```python
from build123d import *

# Parameters (mm, degrees)
SKETCH2_W               = 88.9
SKETCH2_H               = 152.4
BOSS_EXTRUDE1_DEPTH     = 5.9944
CUT_EXTRUDE2_DEPTH      = 177.535840076
CUT_EXTRUDE2_DEPTH_BACK = 177.535840076
SKETCH4_R               = 2.7305
BOSS_EXTRUDE2_DEPTH     = 101.6
FILLET1_R               = 3.81
FILLET2_R               = 2.54
BOSS_EXTRUDE3_DEPTH     = 20.32
FILLET3_R               = 3.81
FILLET6_R               = 3.81
FILLET7_R               = 2.54
CUT_EXTRUDE3_DEPTH      = 204.596488182
CUT_EXTRUDE3_DEPTH_BACK = 204.596488182
SKETCH7_W               = 2.54
SKETCH7_H               = 152.4


with BuildPart() as part:
    # Sketch2 → Boss-Extrude1 (new body)
    with BuildSketch(Plane(origin=(0, 0, 0), x_dir=(1, 0, 0), z_dir=(0, 1, 0))):
        with Locations((44.45, 76.2)):
            Rectangle(SKETCH2_W, SKETCH2_H)
    extrude(amount=BOSS_EXTRUDE1_DEPTH)

    # Sketch4 → Cut-Extrude2 (cut, two sides: drawn at the far end of the back side and taken through both)
    with BuildSketch(Plane(origin=(0, 5.9944, 0), x_dir=(1, 0, 0), z_dir=(0, 1, 0)).offset(-CUT_EXTRUDE2_DEPTH_BACK)):
        with Locations(Location((45.72, 109.871331367, 0), (0, 0, 270))):
            Circle(SKETCH4_R)
        with Locations(Location((45.72, 33.671331367, 0), (0, 0, 270))):
            Circle(SKETCH4_R)
    extrude(amount=CUT_EXTRUDE2_DEPTH + CUT_EXTRUDE2_DEPTH_BACK, mode=Mode.SUBTRACT)

    # Sketch5 → Boss-Extrude2 (add)
    with BuildSketch(Plane(origin=(0, 5.9944, 0), x_dir=(1, 0, 0), z_dir=(0, 1, 0))):
        Polygon((18.542, 15.748), (12.446, 15.748), (12.446, 2.54), (76.454, 2.54), (76.454, 15.748), (70.358, 15.748), (70.358, 13.208), (71.374, 13.208), (71.374, 11.43), (70.358, 11.43), (70.358, 7.62), (18.542, 7.62), (18.542, 11.43), (17.526, 11.43), (17.526, 13.208), (18.542, 13.208), align=None)
    extrude(amount=BOSS_EXTRUDE2_DEPTH)

    # Fillet1
    fillet1_edges = [part.edges().sort_by_distance(p)[0] for p in [
        (12.446, 56.7944, -15.748),
        (12.446, 56.7944, -2.54),
        (76.454, 56.7944, -2.54),
        (76.454, 56.7944, -15.748),
    ]]
    fillet(fillet1_edges, radius=FILLET1_R)

    # Fillet2
    fillet2_edges = [part.edges().sort_by_distance(p)[0] for p in [
        (71.501, 5.9944, -15.748),
        (44.45, 5.9944, -2.54),
        (12.446, 5.9944, -9.144),
        (17.399, 5.9944, -15.748),
        (76.454, 5.9944, -9.144),
        (13.561923164, 5.9944, -3.655923164),
        (13.561923164, 5.9944, -14.632076836),
        (75.338076836, 5.9944, -3.655923164),
        (75.338076836, 5.9944, -14.632076836),
    ]]
    fillet(fillet2_edges, radius=FILLET2_R - 0.0001)  # a hair under: the kernel refuses the full size

    # Sketch6 → Boss-Extrude3 (add, symmetric)
    with BuildSketch(Plane.ZY.offset(-44.45)):
        Polygon((-149.86, 5.9944), (-79.121, 5.9944), (-79.121, 23.1394), (-86.106, 23.1394), (-86.106, 18.0594), (-84.201, 18.0594), (-84.201, 16.1544), (-86.106, 16.1544), (-86.106, 11.0744), (-142.875, 11.0744), (-142.875, 16.1544), (-144.78, 16.1544), (-144.78, 18.0594), (-142.875, 18.0594), (-142.875, 23.1394), (-149.86, 23.1394), align=None)
    extrude(amount=BOSS_EXTRUDE3_DEPTH, both=True)

    # Fillet3
    fillet3_edges = [part.edges().sort_by_distance(p)[0] for p in [
        (44.45, 23.1394, -149.86),
        (44.45, 23.1394, -79.121),
    ]]
    fillet(fillet3_edges, radius=FILLET3_R)

    # Fillet6
    fillet6_edges = [part.edges().sort_by_distance(p)[0] for p in [
        (24.13, 12.6619, -149.86),
        (64.77, 12.6619, -79.121),
        (24.13, 23.1394, -84.5185),
        (24.13, 12.6619, -79.121),
        (64.77, 23.1394, -84.5185),
        (64.77, 12.6619, -149.86),
        (64.77, 23.1394, -144.4625),
        (64.77, 22.023476836, -148.744076836),
        (64.77, 22.023476836, -80.236923164),
        (24.13, 23.1394, -144.4625),
        (24.13, 22.023476836, -148.744076836),
        (24.13, 22.023476836, -80.236923164),
    ]]
    fillet(fillet6_edges, radius=FILLET6_R)

    # Fillet7
    fillet7_edges = [part.edges().sort_by_distance(p)[0] for p in [
        (24.13, 5.9944, -114.4905),
        (64.77, 5.9944, -114.4905),
        (44.45, 5.9944, -79.121),
        (44.45, 5.9944, -149.86),
        (25.245923164, 5.9944, -80.236923164),
        (63.654076836, 5.9944, -80.236923164),
        (63.654076836, 5.9944, -148.744076836),
        (25.245923164, 5.9944, -148.744076836),
    ]]
    fillet(fillet7_edges, radius=FILLET7_R - 0.0001)  # a hair under: the kernel refuses the full size

    # Sketch7 → Cut-Extrude3 (cut, two sides: drawn at the far end of the back side and taken through both)
    with BuildSketch(Plane(origin=(0, 5.9944, 0), x_dir=(1, 0, 0), z_dir=(0, 1, 0)).offset(-CUT_EXTRUDE3_DEPTH_BACK)):
        with Locations((1.27, 76.2)):
            Rectangle(SKETCH7_W, SKETCH7_H)
    extrude(amount=CUT_EXTRUDE3_DEPTH + CUT_EXTRUDE3_DEPTH_BACK, mode=Mode.SUBTRACT)


solid = part.part
```
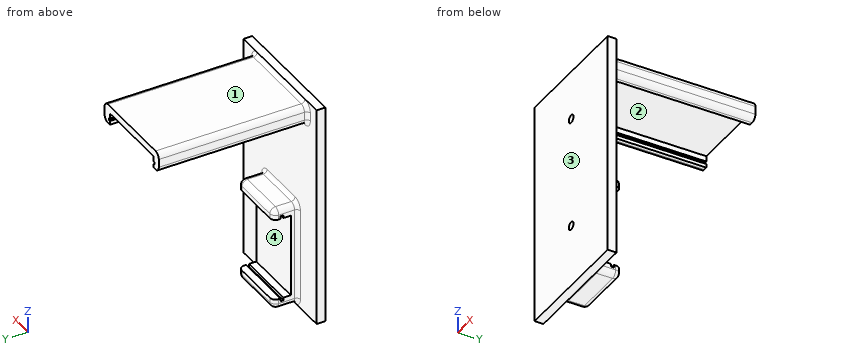
Model file for the job. Use its own axes, mm. Face numbers are marked on the shaded views. A direction names the side the tool comes from. Round coordinates to 2 decimals unless told otherwise and drop trailing zeros. Write each loop counter-clockwise with the first axis right and the second up, starting at its lowest first coordinate (ties: lowest second). Pieces come first, ordered by that corner, then holes. Notation, with made-up numbers: (15.5, 61) -> (55.5, 61) arc R16 ccw to (55.5, 87) -> close; hole circle Ø9 at (-19.5, 54.25). An arc over 180 degrees is marked (long way). Answer as CSV lines item,"result".
1. Slice it at A-A, the plane y = 71. List the corners of the cut face in (x, z).
Resolved:
outline,"(12.45, -11.94) arc R3.81 ccw to (16.26, -15.75) -> (18.54, -15.75) -> (18.54, -13.21) -> (17.53, -13.21) -> (17.53, -11.43) -> (18.54, -11.43) -> (18.54, -7.62) -> (70.36, -7.62) -> (70.36, -11.43) -> (71.37, -11.43) -> (71.37, -13.21) -> (70.36, -13.21) -> (70.36, -15.75) -> (72.64, -15.75) arc R3.81 ccw to (76.45, -11.94) -> (76.45, -6.35) arc R3.81 ccw to (72.64, -2.54) -> (16.26, -2.54) arc R3.81 ccw to (12.45, -6.35) -> close"
2. Mould opens along X. For the marked faces 1 and 2 say: +X half, -X half, draft (parallel to the pull), parting line (faces both ways), or undercut.
Resolved:
face 1,"draft"
face 2,"undercut"
3. Pin check, flat tips, straight feed: pin 1 Ø1.5 at (y, z) = (36, -18) entering from +X; pin 2 Ø6 at (x, z) = (36.5, -99) entering from +Y; pin 3 Ø1 at (x, y) = (35.5, 16.5) entering from +Z; pin 4 Ø3 at (x, y) = (51, 15.5) entering from -Z. Stop position of each tip, or through.
Resolved:
pin 1,"through"
pin 2,"y = 11.07"
pin 3,"z = -2.54"
pin 4,"z = -149.86"
4. Tool access for the marked faces 3 and 4: list every direction of +Z, -Z, +X, -X, +Y, -Y with a clear straight run to the whole face (end or side of a thin tool).
Resolved:
face 3,"+Z, -Z, +X, -X, -Y"
face 4,"+X, -X, +Y"
5. Drill centre lines: line 1 (Z direction, x = 45.72, y = 4.15); line 2 (Z direction, x = 45, y = 3); line 3 (Z direction, x = 18, y = 18.5). Where is each one in solid material? Low to high.
Resolved:
line 1,"-152.4 to -112.6, -107.14 to -36.4, -30.94 to 0"
line 2,"-152.4 to -112.51, -107.24 to -36.31, -31.04 to 0"
line 3,"-15.75 to -13.21, -11.43 to -2.54"
6. Slice it at C-C, the plane z = -51. List the corners of the cut face in (x, y).
Resolved:
outline,"(2.54, 0) -> (88.9, 0) -> (88.9, 5.99) -> (2.54, 5.99) -> close"
7. Slice it at B-B, the plane z = -110. List the corners of the cut face in (x, y), plus the area to 3 significant figures.
Resolved:
outline,"(2.54, 0) -> (42.99, 0) -> (42.99, 5.99) -> (48.45, 5.99) -> (48.45, 0) -> (88.9, 0) -> (88.9, 5.99) -> (67.31, 5.99) arc R2.54 cw to (64.77, 8.53) -> (64.77, 11.07) -> (24.13, 11.07) -> (24.13, 8.53) arc R2.54 cw to (21.59, 5.99) -> (2.54, 5.99) -> close"
area,"694 mm²"
